from build123d import *

# Parameters (mm, degrees)
SKETCH1_R           = 1.905
BOSS_EXTRUDE1_DEPTH = 10.16
SKETCH2_R           = 2.286
CUT_EXTRUDE1_DEPTH  = 20.176579466
FILLET2_R           = 3.81
FILLET1_R           = 1.27


with BuildPart() as part:
    # Sketch1 → Boss-Extrude1 (new body)
    with BuildSketch(Plane(origin=(0, 0, 0), x_dir=(0, 0, -1), z_dir=(1, 0, 0))):
        with BuildLine():
            Line((0, 0), (10.16, 0))
            Line((10.16, 0), (10.16, 12.7))
            Line((10.16, 12.7), (-5.08, 12.7))
            ThreePointArc((-5.08, 12.7), (-10.16, 7.62), (-5.08, 2.54))
            Line((-5.08, 2.54), (0, 2.54))
            Line((0, 2.54), (0, 0))
        make_face()
        with Locations((-5.08, 7.62)):
            Circle(SKETCH1_R, mode=Mode.SUBTRACT)
    extrude(amount=BOSS_EXTRUDE1_DEPTH)

    # Sketch2 → Cut-Extrude1 (cut, through all)
    with BuildSketch(Plane(origin=(0, 12.7, 0), x_dir=(1, 0, 0), z_dir=(0, 1, 0))):
        with Locations(Location((5.08, 5.08, 0), (0, 0, 270))):
            Circle(SKETCH2_R)
    extrude(amount=-CUT_EXTRUDE1_DEPTH, mode=Mode.SUBTRACT)

    # Fillet2
    fillet2_edges = [part.edges().sort_by_distance(p)[0] for p in [
        (10.16, 1.27, 0),
        (0, 1.27, 0),
    ]]
    fillet(fillet2_edges, radius=FILLET2_R)

    # Fillet1
    fillet1_edges = [part.edges().sort_by_distance(p)[0] for p in [
        (5.08, 2.54, 0),
        (1.115923164, 2.54, -1.115923164),
        (9.044076836, 2.54, -1.115923164),
        (5.08, 0, -10.16),
        (5.08, 12.7, -10.16),
    ]]
    fillet(fillet1_edges, radius=FILLET1_R)


solid = part.part
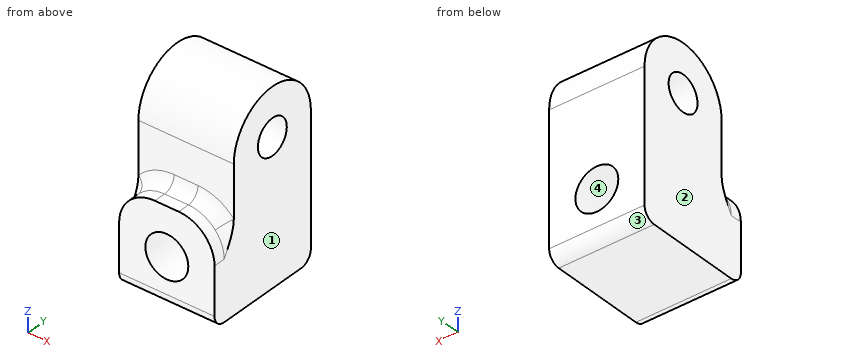
Check sheet for the modelled part. Datum: model origin and axes. Units: mm. Face numbers are marked on the shaded views. Give positions to 0.01 mm unless a question says otherwise; leave off trailing zeros. Write each loop counter-clockwise with the first axis right and the second up, starting at its lowest first coordinate (ties: lowest second). Pieces come first, ordered by that corner, then holes. Notation, with made-up numbers: (-23, 21.5) -> (28, 21.5) arc R32 cw to (28, 53.5) -> close; hole circle Ø5 at (27.5, -2.75). An arc over 180 degrees is marked (long way). Use one line per item in the form item = value. Start each with the question number.
1. Thickness scan on line 1 along X through (y, z) = (4.5, -5.08); line 2 along Z through (x, y) = (5, 1.75); line 3 along X through (y, z) = (9, -6). Record the ranges inside material, lowest first. Write a range as from..to.
2. Go/stop test with flat-tipped pins: P1, Ø1.7, axis at x = 5.5, z = 3, coming from the -Y side; P2, Ø1, axis at y = 7, z = -2, coming from the -X side. Record where each tip stops, or that it passes through.
3. Section check A-A (x = 5.08). Record the cut outline in (y, z) (3 decimals).
4. Section check B-B (y = 7.62). Record the cut outline in (x, z) (3 decimals).
5. Mould release check, pull along X, two halves, no side actions. Record for the marked faces 1, 2, 3 and 4: pulls with the +X half, pulls with the -X half, needs draft (parallel to the pull), parting line crosses it, or undercut.
6. Section check C-C (z = -5.5). Record the cut outline in (x, y), and give its area (3 significant figures).
7. Section check D-D (y = 9.25). Record the cut outline in (x, z).
Conclusion:
q1.line_1 = 0..2.79, 7.37..10.16
q1.line_2 = -10.16..-7.36, -2.8..0.09
q1.line_3 = 0..2.99, 7.17..10.16
q2.P1 = 2.54
q2.P2 = 0
q3.outline = (0, -8.89) arc R1.27 ccw to (1.27, -10.16) -> (11.43, -10.16) arc R1.27 ccw to (12.7, -8.89) -> (12.7, -7.366) -> (0, -7.366) -> close; (0, -2.794) -> (12.7, -2.794) -> (12.7, 5.08) arc R5.08 ccw to (2.54, 5.08) -> (2.54, 1.27) arc R1.27 cw to (1.27, 0) -> (0, 0) -> close; hole circle Ø3.81 at (7.62, 5.08)
q4.outline = (0, -10.16) -> (10.16, -10.16) -> (10.16, 3.175) -> (0, 3.175) -> close; (0, 6.985) -> (10.16, 6.985) -> (10.16, 10.16) -> (0, 10.16) -> close; hole circle Ø4.572 at (5.08, -5.08)
q5.face_1 = pulls with the +X half
q5.face_2 = pulls with the -X half
q5.face_3 = needs draft
q5.face_4 = undercut
q6.outline = (0, 0) -> (2.83, 0) -> (2.83, 12.7) -> (0, 12.7) -> close; (7.33, 0) -> (10.16, 0) -> (10.16, 12.7) -> (7.33, 12.7) -> close
q6.area = 72.0 mm²
q7.outline = (0, -10.16) -> (10.16, -10.16) -> (10.16, 4.09) -> (0, 4.09) -> close; (0, 6.07) -> (10.16, 6.07) -> (10.16, 9.89) -> (0, 9.89) -> close; hole circle Ø4.57 at (5.08, -5.08)
